from build123d import *

# Parameters (mm, degrees)
SKIZZE1_R                       = 1.825
AUFSATZ_LINEAR_AUSTRAGEN1_DEPTH = 10
SCHNITT_LINEAR_AUSTRAGEN1_DEPTH = 2.75
VERRUNDUNG1_R                   = 10
VERRUNDUNG2_R                   = 10
SKIZZE2_R                       = 9
SKIZZE2_R_2                     = 5
AUFSATZ_LINEAR_AUSTRAGEN2_DEPTH = 7.25
AUFSATZ_LINEAR_AUSTRAGEN3_DEPTH = 7.25
KREISMUSTER1_COUNT              = 20
SCHNITT_LINEAR_AUSTRAGEN3_DEPTH = 4
SCHNITT_LINEAR_AUSTRAGEN4_DEPTH = 57.925042167


with BuildPart() as part:
    # Skizze1 → Aufsatz-Linear austragen1 (new body)
    with BuildSketch(Plane(origin=(0, 0, 0), x_dir=(1, 0, 0), z_dir=(0, 1, 0))):
        with BuildLine():
            Line((0, 5), (50, 5))
            ThreePointArc((50, 5), (55, 0), (50, -5))
            Line((50, -5), (0, -5))
            ThreePointArc((0, -5), (-5, 0), (0, 5))
        make_face()
        with Locations(Location((50, 0, 0), (0, 0, 270))):
            Circle(SKIZZE1_R, mode=Mode.SUBTRACT)
        with Locations(Location((0, 0, 0), (0, 0, 270))):
            Circle(SKIZZE1_R, mode=Mode.SUBTRACT)
    extrude(amount=-AUFSATZ_LINEAR_AUSTRAGEN1_DEPTH)

    # Skizze5 → Schnitt-Linear austragen1 (cut)
    with BuildSketch(Plane(origin=(0, 0, 0), x_dir=(1, 0, 0), z_dir=(0, 1, 0))):
        with BuildLine():
            Line((0, -5), (25, -5))
            Line((25, -5), (25, 5))
            Line((25, 5), (0, 5))
            ThreePointArc((0, 5), (-5, 0), (0, -5))
        make_face()
    extrude(amount=-SCHNITT_LINEAR_AUSTRAGEN1_DEPTH, mode=Mode.SUBTRACT)

    # Verrundung1
    # the kernel refuses this fillet: 10 mm, written as the material it adds along each edge
    with BuildSketch(Plane(origin=(25, -2.75, 5), x_dir=(-1, 0, 0), z_dir=(0, 0, -1))) as verrundung1_piece_1:
        with BuildLine():
            CenterArc((6.887488657, 10), VERRUNDUNG1_R, 226.468847833, 43.531152167)
            Line((0, 2.75), (-0.137749773, 2.605))
            ThreePointArc((-0.137749773, 2.605), (-0.2, 1.375), (-0.2, 0))
            Line((-0.2, 0), (0, -0.2))
            Line((0, -0.2), (6.887488657, -0.2))
            Line((6.887488657, -0.2), (6.887488657, 0))
        make_face()
    extrude(amount=10)

    # Verrundung2
    verrundung2_edges = [part.edges().sort_by_distance(p)[0] for p in [
        (25, 0, 0),
    ]]
    fillet(verrundung2_edges, radius=VERRUNDUNG2_R)

    # Skizze2 → Aufsatz-Linear austragen2 (add)
    with BuildSketch(Plane(origin=(0, -2.75, 0), x_dir=(1, 0, 0), z_dir=(0, 1, 0))):
        Circle(SKIZZE2_R)
        Circle(SKIZZE2_R_2, mode=Mode.SUBTRACT)
    extrude(amount=-AUFSATZ_LINEAR_AUSTRAGEN2_DEPTH)

    # Skizze3 → Aufsatz-Linear austragen3 (add)
    with BuildSketch(Plane(origin=(0, -2.75, 0), x_dir=(1, 0, 0), z_dir=(0, 1, 0))):
        with BuildLine():
            Line((-8.979155186, 0.612186368), (-10.745251311, 1.195648052))
            Line((-10.745251311, 1.195648052), (-10.588816846, 2.183336393))
            Line((-10.588816846, 2.183336393), (-8.728860042, 2.192487713))
            ThreePointArc((-8.728860042, 2.192487713), (-8.889195065, 1.407910185), (-8.979155186, 0.612186368))
        make_face()
    aufsatz_linear_austragen3 = extrude(amount=-AUFSATZ_LINEAR_AUSTRAGEN3_DEPTH)

    # Kreismuster1: Aufsatz-Linear austragen3 ×20 about axis
    kreismuster1_axis = Axis((0, 0, 0), (0, 1, 0))
    for i in range(1, KREISMUSTER1_COUNT):
        add(aufsatz_linear_austragen3.rotate(kreismuster1_axis, i * 360 / KREISMUSTER1_COUNT))

    # Skizze8 → Schnitt-Linear austragen3 (cut)
    with BuildSketch(Plane(origin=(0, -2.75, 0), x_dir=(1, 0, 0), z_dir=(0, 1, 0))):
        Polygon((0, 3.175426481), (-2.75, 1.58771324), (-2.75, -1.58771324), (0, -3.175426481), (2.75, -1.58771324), (2.75, 1.58771324), align=None)
    extrude(amount=-SCHNITT_LINEAR_AUSTRAGEN3_DEPTH, mode=Mode.SUBTRACT)

    # Skizze10 → Schnitt-Linear austragen4 (cut, through all)
    with BuildSketch(Plane.XZ.offset(10)):
        with BuildLine():
            Line((9, 3), (31, 3))
            ThreePointArc((31, 3), (34, 0), (31, -3))
            Line((31, -3), (9, -3))
            ThreePointArc((9, -3), (6, 0), (9, 3))
        make_face()
    extrude(amount=-SCHNITT_LINEAR_AUSTRAGEN4_DEPTH, mode=Mode.SUBTRACT)


solid = part.part
Input: part model. Units: mm. Frame: model coordinates. A direction names the side the tool comes from. Coordinates: 2 decimals unless noted, no trailing zeros. Loops run counter-clockwise (first coordinate to the right, second up) from the corner with the lowest first, then second, coordinate; pieces in that order, holes last.
(1) Set-up query: faces 1 (the face through (1.394, -4.722, -2.37)), 2 (the face through (5.07, -6.32, -8.52)), 3 (the face through (-9.111, -6.324, 3.915)). Return all of +Z, -Z, +X, -X, +Y, -Y with unobstructed straight access to the full face (end or side cutting, diameter ignored); none if empty.
(2) Section B-B on x = 15.5. Return the cut outline in (y, z), then the cut area to 3 significant figures.
(3) Pull-direction query (Z, two-part tool) for faces 4 (the face through (-7.44, -6.32, -6.52)), 5 (the face through (6.52, -6.32, -7.44)), 6 (the face through (42, 0, 0)), 7 (the face through (-3.9, -6.32, 9.09)); classes: released by +Z, released by -Z, zero draft, split by the parting line, or undercut.
(4) Material intervals for probe 1 along X at (y, z) = (-3, 0) (3 decimals); probe 2 along X at (y, z) = (-9.3, 0) (3 decimals); probe 3 along X at (y, z) = (-2, 0) (3 decimals), sorted ascending.
(5) Section D-D on x = 30. Return the cut outline in (y, z), then the cut area to 3 significant figures.
(6) Section C-C on y = -2. Return the cut outline in (x, z) (3 decimals).
(7) Section A-A on z = 0. Return the cut outline in (x, y) (3 decimals).
(8) First-contact query: pin 1 Ø0.7 at (x, y) = (8, -8) entering from -Z; pin 2 Ø3 at (x, y) = (19, -6) entering from -Z; pin 3 Ø4 at (y, z) = (-5.5, -5) entering from -X. Flat tips, straight axial feed; report the tip coordinate or a pass-through.
Data:
1. face 1: +Y
1. face 2: +Y, -Y
1. face 3: -X, +Y, -Y
2. outline: (-10, -5) - (-2.75, -5) - (-2.75, -3) - (-10, -3) - close; (-10, 3) - (-2.75, 3) - (-2.75, 5) - (-10, 5) - close
2. area: 29.0 mm2
3. face 4: undercut
3. face 5: released by -Z
3. face 6: zero draft
3. face 7: released by +Z
4. probe 1: x = -9 to -2.75, 2.75 to 6, 34 to 48.175, 51.825 to 55
4. probe 2: x = -9 to -1.825, 1.825 to 6, 34 to 48.175, 51.825 to 55
4. probe 3: x = 34 to 48.175, 51.825 to 55
5. outline: (-10, -5) - (0, -5) - (0, -3) - (-10, -3) - close; (-10, 3) - (0, 3) - (0, 5) - (-10, 5) - close
5. area: 40.0 mm2
6. outline: (21.912, -5) - (50, -5) arc R5 ccw to (50, 5) - (21.912, 5) - (21.912, 3) - (31, 3) arc R3 cw to (31, -3) - (21.912, -3) - close; hole circle Ø3.65 at (50, 0)
7. outline: (-9, -10) - (-1.825, -10) - (-1.825, -6.75) - (-2.75, -6.75) - (-2.75, -2.75) - (-9, -2.75) - close; (1.825, -10) - (6, -10) - (6, -2.75) - (2.75, -2.75) - (2.75, -6.75) - (1.825, -6.75) - close; (34, -10) - (48.175, -10) - (48.175, 0) - (34, 0) - close; (51.825, -10) - (55, -10) - (55, 0) - (51.825, 0) - close
8. pin 1: stops at z = -7.62
8. pin 2: stops at z = -5
8. pin 3: stops at x = -9.85
